```python
from build123d import *

# Parameters (mm, degrees)
SKETCH1_R           = 6
BOSS_EXTRUDE1_DEPTH = 10
SKETCH2_R           = 1.025
CUT_EXTRUDE1_DEPTH  = 7
SKETCH4_R           = 2.275
CUT_EXTRUDE4_DEPTH  = 11.0000001
SKETCH5_W           = 0.95
SKETCH5_H           = 7.069146706
BOSS_EXTRUDE2_DEPTH = 1.2
SKETCH7_R           = 6
BOSS_EXTRUDE3_DEPTH = 1
SKETCH8_R           = 2.625
SKETCH8_W           = 2.25
SKETCH8_H           = 1.25
BOSS_EXTRUDE4_DEPTH = 6.5
SKETCH9_R           = 1.075
CUT_EXTRUDE5_DEPTH  = 6
CUT_EXTRUDE2_START  = -3
CUT_EXTRUDE2_DEPTH  = 2.2


with BuildPart() as part:
    # Sketch1 → Boss-Extrude1 (new body)
    with BuildSketch(Plane(origin=(0, 0, 0), x_dir=(1, 0, 0), z_dir=(0, 1, 0))):
        Circle(SKETCH1_R)
    extrude(amount=BOSS_EXTRUDE1_DEPTH)

    # Sketch2 → Cut-Extrude1 (cut, through all)
    with BuildSketch(Plane.XY):
        with Locations((0, 7)):
            Circle(SKETCH2_R)
    extrude(amount=-CUT_EXTRUDE1_DEPTH, mode=Mode.SUBTRACT)

    # Sketch4 → Cut-Extrude4 (cut, through all)
    with BuildSketch(Plane(origin=(0, 0, 0), x_dir=(1, 0, 0), z_dir=(0, 1, 0))):
        Circle(SKETCH4_R)
    extrude(amount=CUT_EXTRUDE4_DEPTH, mode=Mode.SUBTRACT)

    # Sketch5 → Boss-Extrude2 (add)
    with BuildSketch(Plane(origin=(0, 10, 0), x_dir=(1, 0, 0), z_dir=(0, 1, 0))):
        Rectangle(SKETCH5_W, SKETCH5_H)
    extrude(amount=-BOSS_EXTRUDE2_DEPTH)

    # Sketch7 → Boss-Extrude3 (add)
    with BuildSketch(Plane(origin=(0, 10, 0), x_dir=(1, 0, 0), z_dir=(0, 1, 0))):
        Circle(SKETCH7_R)
    extrude(amount=BOSS_EXTRUDE3_DEPTH)

    # Sketch8 → Boss-Extrude4 (add)
    with BuildSketch(Plane(origin=(0, 11, 0), x_dir=(1, 0, 0), z_dir=(0, 1, 0))):
        Circle(SKETCH8_R)
        with Locations((0, -2.625)):
            Rectangle(SKETCH8_W, SKETCH8_H)
    extrude(amount=BOSS_EXTRUDE4_DEPTH)

    # Sketch9 → Cut-Extrude5 (cut)
    with BuildSketch(Plane(origin=(0, 17.5, 0), x_dir=(1, 0, 0), z_dir=(0, 1, 0))):
        Circle(SKETCH9_R)
    extrude(amount=-CUT_EXTRUDE5_DEPTH, mode=Mode.SUBTRACT)

    # Sketch3 → Cut-Extrude2 (cut)
    with BuildSketch(Plane.XY.offset(CUT_EXTRUDE2_START)):
        Polygon((0, 4.401923789), (2.25, 5.700961894), (2.25, 8.299038106), (2.25, 11.472802467), (-2.25, 11.472802467), (-2.25, 8.299038106), (-2.25, 5.700961894), align=None)
    extrude(amount=-CUT_EXTRUDE2_DEPTH, mode=Mode.SUBTRACT)


solid = part.part
```
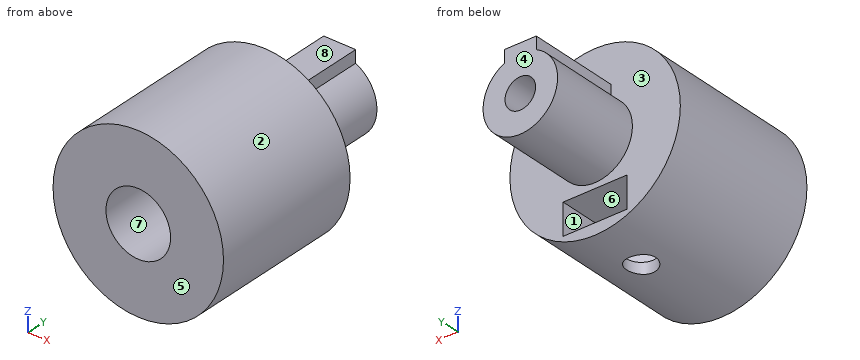
CAD build for the part. Positions are in the model's coordinates, mm. Face numbers are marked on the shaded views. A direction names the side the tool comes from. Round coordinates to 2 decimals unless told otherwise and drop trailing zeros. Write each loop counter-clockwise with the first axis right and the second up, starting at its lowest first coordinate (ties: lowest second). Pieces come first, ordered by that corner, then holes.
Item 1: Mould opens along X. For the marked faces 1, 2 and 3 say: released by +X, released by -X, zero draft, split by the parting line, or undercut.
Filled in:
face 1: undercut
face 2: split by the parting line
face 3: zero draft
Item 2: Drop flat-ended pins along their axis: pin 1 Ø1.6 at (x, y) = (0, 7) entering from -Z; pin 2 Ø1.3 at (x, z) = (0, 0) entering from -Y; pin 3 Ø2 at (x, y) = (3, 6) entering from -Z. Give the stop position or say it passes through.
Filled in:
pin 1: stops at z = 2.13
pin 2: stops at y = 8.8
pin 3: stops at z = -5.66
Item 3: Drill centre lines: L1, parallel to Z at x = 0, y = 2.25 (3 decimals); L2, parallel to Y at x = 0, z = -5.75 (3 decimals); L3, parallel to Z at x = -1, y = 9.75. Where is each one in solid material? Low to high.
Filled in:
L1: z = -6 to -2.275, 2.275 to 6
L2: y = 0 to 5.975, 8.025 to 11
L3: z = -5.92 to -5.2, -3 to -2.04, 2.04 to 5.92
Item 4: Tool access for the marked faces 4, 5, 6, 7 and 8: list every direction of +Z, -Z, +X, -X, +Y, -Y with a clear straight run to the whole face (end or side of a thin tool).
Filled in:
face 4: +Z, -Z, +X, -X, +Y
face 5: +Z, -Z, +X, -X, -Y
face 6: +Y
face 7: -Y
face 8: +Z, +X, -X, +Y
Item 5: Band-saw the part on D-D on y = 7. Write the cut outline in (x, z) (3 decimals), then the cut area to 3 significant figures.
Filled in:
outline: (-2.25, -5.2) - (-2.25, -3) - (-1.025, -3) - (-1.025, -2.031) arc R2.275 cw (long way) to (1.025, -2.031) - (1.025, -3) - (2.25, -3) - (2.25, -5.2) - (1.025, -5.2) - (1.025, -5.912) arc R6 ccw (long way) to (-1.025, -5.912) - (-1.025, -5.2) - close
area: 83.7 mm2
Item 6: Band-saw the part on A-A on y = 10.5. Write the cut outline in (x, z).
Filled in:
outline: circle Ø12 at (0, 0); hole (-2.25, -5.2) - (2.25, -5.2) - (2.25, -3) - (-2.25, -3) - close
Item 7: Band-saw the part on B-B on z = -4.25. Write the cut outline in (x, y).
Filled in:
outline: (-4.24, 0) - (4.24, 0) - (4.24, 11) - (2.25, 11) - (2.25, 5.7) - (0, 4.4) - (-2.25, 5.7) - (-2.25, 11) - (-4.24, 11) - close
Item 8: Band-saw the part on C-C on y = 14.5. Write the cut outline in (x, z) (3 decimals), then the cut area to 3 significant figures.
Filled in:
outline: (-1.125, 2.372) arc R2.625 ccw (long way) to (1.125, 2.372) - (1.125, 3.25) - (-1.125, 3.25) - close; hole circle Ø2.15 at (0, 0)
area: 19.6 mm2
